from build123d import *

# Parameters (mm, degrees)
F0_R     = 5
F2_R     = 10
F5_DEPTH = 5.08
F6_DEPTH = 5.08


with BuildPart() as f3:
    # F0 (on Top) → F3 section 0
    with BuildSketch(Plane.XY):
        Circle(F0_R)
    # F2 (on offset) → F3 section 1
    with BuildSketch(Plane.XY.offset(25.4)):
        Circle(F2_R)
    loft()

    # F4 (on Front) → F5 (join)
    with BuildSketch(Plane.XZ):
        with BuildLine():
            ThreePointArc((17.960512, 37.010512), (17.960512, 54.971024), (0, 54.971024))
            ThreePointArc((0, 54.971024), (-17.960512, 54.971024), (-17.960512, 37.010512))
            Line((-17.960512, 37.010512), (0, 19.05))
            Line((0, 19.05), (17.960512, 37.010512))
        make_face()
    extrude(amount=F5_DEPTH)

    # F4 (on Front) → F6 (join)
    with BuildSketch(Plane.XZ):
        with BuildLine():
            ThreePointArc((17.960512, 37.010512), (17.960512, 54.971024), (0, 54.971024))
            ThreePointArc((0, 54.971024), (-17.960512, 54.971024), (-17.960512, 37.010512))
            Line((-17.960512, 37.010512), (0, 19.05))
            Line((0, 19.05), (17.960512, 37.010512))
        make_face()
    extrude(amount=-F6_DEPTH)


solid = f3.part
The model under review builds one solid part; all positions refer to its coordinate system, in mm. A direction names the side the tool comes from. Coordinates: 2 decimals unless noted, no trailing zeros. Order: outer loops, then holes, each group sorted by start corner. A loop starts at its lowest first (then second) coordinate and runs counter-clockwise, first axis right, second up. Notation, with made-up numbers: (71, -3.75) -> (99, -3.75) arc R16 ccw to (99, 2.25) -> close; hole circle Ø5 at (1, 72). An arc over 180 degrees is marked (long way). Answer in a Markdown table with one row per item.
(1) Wall thickness on line 1 along Y through (x, z) = (-13, 32.5); line 2 along X through (y, z) = (-4, 45.5); line 3 along Z through (x, y) = (-11, -3): over which ranges is each line inside the solid? List them lowest first.
Answers:
| item | result |
|---|---|
| line 1 | -5.08 to 5.08 |
| line 2 | -21.67 to 21.67 |
| line 3 | 30.05 to 58.53 |
(2) Consider section B-B (x = 14). Write out the cut boundary in (y, z).
Answers:
| item | result |
|---|---|
| outline | (-5.08, 33.05) -> (5.08, 33.05) -> (5.08, 57.66) -> (-5.08, 57.66) -> close |
(3) The part is to be moulded in two halves that separate along X. For faces 1 (the flat face through (12.07, -0.07, 31.12)), 2 (the cylindrical face through (18.156, -0.071, 54.771)), 3 (the flat face through (0, 0, 0)), say which applies: +X half, -X half, draft (parallel to the pull), parting line (faces both ways), or undercut.
Answers:
| item | result |
|---|---|
| face 1 | +X half |
| face 2 | undercut |
| face 3 | draft |
(4) Machinability: for faces 4 (the flat face through (0, 5.08, 42)), 5 (the flat face through (7, 0, 25.4)), 6 (the flat face through (-12.24, -0.07, 31.29)), which of the approach directions +Z, -Z, +X, -X, +Y, -Y give a long, thin tool a straight path to every point of the face, cutting with its end or side? Answer none if there is none.
Answers:
| item | result |
|---|---|
| face 4 | +Z, +X, -X, +Y |
| face 5 | none |
| face 6 | -X, +Y, -Y |
(5) Insertion check: pin 1 (8 mm diameter, centred on y = -5, z = 29, fed in from +X); pin 2 (16.5 mm diameter, centred on x = 1, z = 38, fed in from -Y); pin 3 (8 mm diameter, centred on y = 8, z = 18, fed in from +X). Each pin has a flat end and moves straight along its axis. Give the tip position at first contact, or say it passes through.
Answers:
| item | result |
|---|---|
| pin 1 | x = 13.95 |
| pin 2 | y = -5.08 |
| pin 3 | x = 7.73 |
(6) Consider section C-C (z = 15.5). Write out the cut boundary in (x, y), plus the area to 3 significant figures.
Answers:
| item | result |
|---|---|
| outline | circle Ø16.1 at (0, 0) |
| area | 204 mm² |
(7) Consider section D-D (z = 4). Write out the cut boundary in (x, y).
Answers:
| item | result |
|---|---|
| outline | circle Ø11.57 at (0, 0) |
(8) Consider section A-A (z = 36). Write out the cut boundary in (x, y).
Answers:
| item | result |
|---|---|
| outline | (-16.95, -5.08) -> (16.95, -5.08) -> (16.95, 5.08) -> (-16.95, 5.08) -> close |
